```python
from build123d import *

# Parameters (mm, degrees)
SKETCH067_W     = 56
SKETCH067_H     = 56
SKETCH067_R     = 2.5
SKETCH067_R_2   = 13
PAD053_DEPTH    = 30
SKETCH068_R     = 10
POCKET007_DEPTH = 14
SKETCH069_R     = 2.65
POCKET008_DEPTH = 7
SKETCH070_R     = 10
POCKET009_DEPTH = 14
SKETCH071_R     = 20
POCKET010_DEPTH = 1.6


with BuildPart() as part:
    # Sketch067 → Pad053 (new body)
    with BuildSketch(Plane.YZ):
        Rectangle(SKETCH067_W, SKETCH067_H)
        with Locations((-23.5, 23.5)):
            Circle(SKETCH067_R, mode=Mode.SUBTRACT)
        with Locations((23.5, 23.5)):
            Circle(SKETCH067_R, mode=Mode.SUBTRACT)
        with Locations((23.5, -23.5)):
            Circle(SKETCH067_R, mode=Mode.SUBTRACT)
        with Locations((-23.5, -23.5)):
            Circle(SKETCH067_R, mode=Mode.SUBTRACT)
        Circle(SKETCH067_R_2, mode=Mode.SUBTRACT)
    extrude(amount=PAD053_DEPTH)

    # Sketch068 (on Face4 of Pad053) → Pocket007 (cut)
    with BuildSketch(Plane(origin=(0, -28, 0), x_dir=(0, 0, -1), z_dir=(0, -1, 0))):
        with Locations((8, 15)):
            Circle(SKETCH068_R)
    extrude(amount=-POCKET007_DEPTH, mode=Mode.SUBTRACT)

    # Sketch069 (on Face5 of Pocket007) → Pocket008 (cut)
    with BuildSketch(Plane.YZ.offset(30)):
        with Locations((-20.5, -8)):
            Circle(SKETCH069_R)
        with Locations((20.5, -8)):
            Circle(SKETCH069_R)
    extrude(amount=-POCKET008_DEPTH, mode=Mode.SUBTRACT)

    # Sketch070 (on Face3 of Pocket008) → Pocket009 (cut)
    with BuildSketch(Plane.ZX.offset(28)):
        with Locations((-8, 15)):
            Circle(SKETCH070_R)
    extrude(amount=-POCKET009_DEPTH, mode=Mode.SUBTRACT)

    # Sketch071 (on Face4 of Pocket009) → Pocket010 (cut)
    with BuildSketch(Plane(origin=(0, 0, 0), x_dir=(0, 1, 0), z_dir=(-1, 0, 0))):
        Circle(SKETCH071_R)
    extrude(amount=-POCKET010_DEPTH, mode=Mode.SUBTRACT)


with BuildPart() as part_1:
    # Body040 placement: moved
    add(part.part.moved(Location((-15, 0, 8))))


solid = part_1.part
```
The model under review builds one solid part; all positions refer to its coordinate system, in mm. A direction names the side the tool comes from. Give positions to 0.01 mm unless a question says otherwise; leave off trailing zeros. Write each loop counter-clockwise with the first axis right and the second up, starting at its lowest first coordinate (ties: lowest second). Pieces come first, ordered by that corner, then holes.
(1) Tool access review of faces 1 (the cylindrical face through (-9.76, 21.1, -2.17)), 2 (the cylindrical face through (12.352, -19.277, -2.351)), 3 (the flat face through (-13.4, 13, 12)): name each direction out of +Z, -Z, +X, -X, +Y, -Y from which nothing blocks a thin tool from reaching the whole face with its end or side.
(2) To check wall thickness, follow L1, parallel to Z at x = -11, y = 23.5; L2, parallel to Y at x = -8.5, z = 8.5; L3, parallel to Y at x = -3, z = -15. State the ranges of each line that lie inside material, in increasing order.
(3) Consider section C-C, the plane y = 0. Give the boundary of the cut face in (x, z), and give its area (3 significant figures).
(4) Consider section D-D, the plane z = -15.5. Give the boundary of the cut face in (x, y), and give its area (3 significant figures).
(5) For P1, Ø3, axis at y = -23.5, z = -15.5, coming from the +X side; P2, Ø10, axis at x = -3, z = 2.5, coming from the -Y side; P3, Ø4, axis at y = 20.5, z = 0, coming from the +X side, all flat-tipped, find the tip position at first contact; note any pin that passes through.
(6) The part is to be moulded in two halves that separate along Z. For faces 4 (the flat face through (15, -7, 21)), 5 (the flat face through (0, 0, 36)), 6 (the flat face through (0, -14, 0)), say which applies: released by +Z, released by -Z, zero draft, split by the parting line, or undercut.
(7) Consider section A-A, the plane z = 8. Give the boundary of the cut face in (x, y).
(8) Consider section B-B, the plane x = 0. Give the boundary of the cut face in (y, z), and give its area (3 significant figures).
Returned:
1. face 1: +Y
1. face 2: +X
1. face 3: -X
2. L1: z = -20 to -18, -13 to 29, 34 to 36
2. L2: y = -28 to -12.99, 12.99 to 28
2. L3: y = -28 to -25.95, -21.05 to 21.05, 25.95 to 28
3. outline: (-15, -20) - (15, -20) - (15, -5) - (-13.4, -5) - (-13.4, -12) - (-15, -12) - close; (-15, 28) - (-13.4, 28) - (-13.4, 21) - (15, 21) - (15, 36) - (-15, 36) - close
3. area: 878 mm2
4. outline: (-15, -28) - (15, -28) - (15, -26) - (-15, -26) - close; (-15, -21) - (15, -21) - (15, 21) - (-15, 21) - close; (-15, 26) - (15, 26) - (15, 28) - (-15, 28) - close
4. area: 1,380 mm2
5. P1: passes through
5. P2: stops at y = -14
5. P3: stops at x = -9.8
6. face 4: zero draft
6. face 5: released by +Z
6. face 6: undercut
7. outline: (-15, -28) - (-6, -28) - (-6, -14) - (6, -14) - (6, -28) - (15, -28) - (15, -13) - (-13.4, -13) - (-13.4, -20) - (-15, -20) - close; (-15, 20) - (-13.4, 20) - (-13.4, 13) - (15, 13) - (15, 28) - (6, 28) - (6, 14) - (-6, 14) - (-6, 28) - (-15, 28) - close
8. outline: (-28, -20) - (28, -20) - (28, -10) - (14, -10) - (14, 10) - (28, 10) - (28, 36) - (-28, 36) - (-28, 10) - (-14, 10) - (-14, -10) - (-28, -10) - close; hole circle Ø5 at (-23.5, -15.5); hole circle Ø5 at (-23.5, 31.5); hole circle Ø26 at (0, 8); hole circle Ø5 at (23.5, -15.5); hole circle Ø5 at (23.5, 31.5)
8. area: 1,970 mm2
